```python
from build123d import *

# Parameters (mm, degrees)
BOSS_EXTRUDE1_DEPTH     = 90
BOSS_EXTRUDE2_START     = -30
SKETCH2_3_R             = 12.5
BOSS_EXTRUDE2_DEPTH     = 60
EXTRUDE_THIN1_DEPTH     = 115
SKETCH5_W               = 50
SKETCH5_H               = 20
BOSS_EXTRUDE3_DEPTH     = 230
CUT_EXTRUDE2_DEPTH      = 315.682379551
CUT_EXTRUDE2_DEPTH_BACK = 315.682379551
SKETCH5_3_R             = 5
CUT_EXTRUDE1_START      = -30
CUT_EXTRUDE1_OUTLINE_R  = 8.5
CUT_EXTRUDE1_DEPTH      = 120
RIB1_START              = -2.5
RIB1_DEPTH              = 5
FILLET1_R               = 10


# Read off the part's stored shape, not the designer's step: Cut-Extrude1, Rib1
with BuildPart() as part:
    # Sketch2 → Boss-Extrude1 (new body)
    with BuildSketch(Plane(origin=(0, 0, 0), x_dir=(1, 0, 0), z_dir=(0, 1, 0))):
        with BuildLine():
            Line((42.074338973, 6), (47.5, 6))
            Line((47.5, 6), (47.5, -6))
            Line((47.5, -6), (42.074338973, -6))
            ThreePointArc((42.074338973, -6), (-42.5, 0), (42.074338973, 6))
        make_face()
    extrude(amount=BOSS_EXTRUDE1_DEPTH)



with BuildPart() as body_2:
    # Sketch2<3> → Boss-Extrude2 (new body)
    with BuildSketch(Plane(origin=(0, 0, 0), x_dir=(1, 0, 0), z_dir=(0, 1, 0)).offset(BOSS_EXTRUDE2_START)):
        with Locations(Location((170, 0, 0), (0, 0, 270))):
            Circle(SKETCH2_3_R)
    extrude(amount=BOSS_EXTRUDE2_DEPTH)


with BuildPart() as part_1:
    add(part.part)

    add(body_2.part)  # Extrude-Thin1 merges body 2
    # Sketch3 → Extrude-Thin1 (add, symmetric)
    with BuildSketch(Plane.XY):
        Polygon((-42.5, 0), (94.247392222, 0), (130, -30), (182.5, -30), (182.5, -24), (132.183821406, -24), (96.431213628, 6), (-42.5, 6), align=None)
    extrude(amount=EXTRUDE_THIN1_DEPTH, both=True)

    # Sketch5 → Boss-Extrude3 (add)
    with BuildSketch(Plane.XY.offset(115)):
        with Locations((170, -20)):
            Rectangle(SKETCH5_W, SKETCH5_H)
    extrude(amount=-BOSS_EXTRUDE3_DEPTH)

    # Sketch5<3> → Cut-Extrude2 (cut, two sides: drawn at the far end of the back side and taken through both)
    with BuildSketch(Plane.XY.offset(115).offset(-CUT_EXTRUDE2_DEPTH_BACK)):
        with Locations((155, -20)):
            Circle(SKETCH5_3_R)
    extrude(amount=CUT_EXTRUDE2_DEPTH + CUT_EXTRUDE2_DEPTH_BACK, mode=Mode.SUBTRACT)

    # Cut-Extrude1 outline → Cut-Extrude1 (cut)
    with BuildSketch(Plane(origin=(0, 0, 0), x_dir=(1, 0, 0), z_dir=(0, 1, 0)).offset(CUT_EXTRUDE1_START)):
        with BuildLine():
            ThreePointArc((-42.5, 2.03e-07), (-27.271780209, 32.596012091), (7.5, 41.833001327))
            Line((7.5, 41.833001327), (145, 17.181411259))
            Line((145, 17.181411259), (145, 115))
            Line((145, 115), (-42.5, 115))
            Line((-42.5, 115), (-42.5, 2.03e-07))
        make_face()
        with BuildLine():
            Line((145, 115), (145, 17.181411259))
            Line((145, 17.181411259), (172.205882353, 12.30382392))
            ThreePointArc((172.205882353, 12.30382392), (179.587062361, 8.021111849), (182.5, 0))
            ThreePointArc((182.5, 0), (179.587062361, -8.021111849), (172.205882353, -12.30382392))
            Line((172.205882353, -12.30382392), (145, -17.181411259))
            Line((145, -17.181411259), (145, -115))
            Line((145, -115), (195, -115))
            Line((195, -115), (195, 115))
            Line((195, 115), (145, 115))
        make_face()
        with BuildLine():
            ThreePointArc((7.5, -41.833001327), (-27.271780365, -32.596011961), (-42.5, 2.03e-07))
            Line((-42.5, 2.03e-07), (-42.5, -115))
            Line((-42.5, -115), (145, -115))
            Line((145, -115), (145, -17.181411259))
            Line((145, -17.181411259), (7.5, -41.833001327))
        make_face()
        with BuildLine():
            Line((44.5, 3), (38.382938918, 3))
            ThreePointArc((38.382938918, 3), (-38.5, 0), (38.382938918, -3))
            Line((38.382938918, -3), (44.5, -3))
            Line((44.5, -3), (44.5, 3))
        make_face()
        with Locations((170, 0)):
            Circle(CUT_EXTRUDE1_OUTLINE_R)
    extrude(amount=CUT_EXTRUDE1_DEPTH, mode=Mode.SUBTRACT)

    # Rib1 outline → Rib1 (add)
    with BuildSketch(Plane.XY.offset(RIB1_START)):
        Polygon((151.838214056, 30), (80.3329985, 90), (47.5, 90), (47.5, 6), (96.431213628, 6), (132.183821406, -24), (145, -24), (145, -10), (159, -10), (159, 30), align=None)
    extrude(amount=RIB1_DEPTH)

    # Fillet1
    fillet1_edges = [part_1.edges().sort_by_distance(p)[0] for p in [
        (145, -10, 9.84070563),
        (132.183821406, -24, -10.989575378),
        (96.431213628, 6, -14.194515854),
        (151.838214056, 30, 0),
        (80.3329985, 90, 0),
        (145, -10, -9.84070563),
        (94.247392222, 0, 0),
        (96.431213628, 6, 14.194515854),
        (132.183821406, -24, 10.989575378),
        (130, -30, 0),
    ]]
    fillet(fillet1_edges, radius=FILLET1_R)


solid = part_1.part
```
Source: CAD feature listing. Evaluate the final solid. Frame: model axes, mm. A direction names the side the tool comes from. Give positions to 0.01 mm unless a question says otherwise; leave off trailing zeros. Order: outer loops, then holes, each group sorted by start corner. A loop starts at its lowest first (then second) coordinate and runs counter-clockwise, first axis right, second up. Notation, with made-up numbers: (68, 31.5) -> (101, 31.5) arc R14 ccw to (101, 40.5) -> close; hole circle Ø3 at (3.5, 21). An arc over 180 degrees is marked (long way). Use a Markdown table: item, result.
Q1. Section B-B (y = 26). Return the cut outline in (x, z).
A:
| item | result |
|---|---|
| outline | (42.07, -6) -> (47.5, -6) -> (47.5, -2.5) -> (157.75, -2.5) arc R12.5 ccw (long way) to (157.75, 2.5) -> (47.5, 2.5) -> (47.5, 6) -> (42.07, 6) arc R42.5 ccw (long way) to start; hole (38.38, -3) -> (44.5, -3) -> (44.5, 3) -> (38.38, 3) arc R38.5 ccw (long way) to start; hole circle Ø17 at (170, 0) |
Q2. Section A-A (z = 0). Return the cut outline in (x, y), and give its area (3 significant figures).
A:
| item | result |
|---|---|
| outline | (-42.5, 0) -> (-38.5, 0) -> (-38.5, 90) -> (-42.5, 90) -> close; (44.5, 0) -> (90.61, 0) arc R10 cw to (97.04, -2.34) -> (127.21, -27.66) arc R10 ccw to (133.64, -30) -> (161.5, -30) -> (161.5, 30) -> (155.48, 30) arc R10 cw to (149.05, 32.34) -> (83.12, 87.66) arc R10 ccw to (76.69, 90) -> (44.5, 90) -> close; (178.5, -30) -> (182.5, -30) -> (182.5, 30) -> (178.5, 30) -> close; hole circle Ø10 at (155, -20) |
| area | 9,810 mm^2 |
Q3. Access query for faces 1 (the face through (41, 44, -3)), 2 (the face through (140, -24, 11)), 3 (the face through (114.52, -9.18, -13.78)). Directions: +Z, -Z, +X, -X, +Y, -Y. A direction counts if a zero-diameter tool reaches every point of the face in a straight line with its end or side. Return the directions, or none.
A:
| item | result |
|---|---|
| face 1 | +Y, -Y |
| face 2 | +Z, +Y |
| face 3 | -Z, +Y |
Q4. Section D-D (z = -31). Return the cut outline in (x, y), and give its area (3 significant figures).
A:
| item | result |
|---|---|
| outline | (-29.07, 0) -> (-22.83, 0) -> (-22.83, 90) -> (-29.07, 90) -> close; (22.83, 0) -> (67.92, 0) -> (67.92, 6) -> (29.07, 6) -> (29.07, 90) -> (22.83, 90) -> close |
| area | 1,360 mm^2 |
Q5. Material intervals for line 1 (X direction, y = 0.5, z = 0); line 2 (Z direction, x = 170, y = 6); line 3 (X direction, y = -23, z = 2), sorted ascending. Write a range as [from, to].
A:
| item | result |
|---|---|
| line 1 | [-42.5, -38.5], [44.5, 161.5], [178.5, 182.5] |
| line 2 | [-12.5, -8.5], [8.5, 12.5] |
| line 3 | [121.66, 151], [159, 161.74], [178.26, 182.34] |
Q6. Section C-C (x = 0). Return the cut outline in (y, z), and give its area (3 significant figures).
A:
| item | result |
|---|---|
| outline | (0, -42.5) -> (90, -42.5) -> (90, -38.5) -> (0, -38.5) -> close; (0, 38.5) -> (90, 38.5) -> (90, 42.5) -> (0, 42.5) -> close |
| area | 720 mm^2 |
Q7. Pull-direction query (Z, two-part tool) for faces 4 (the face through (-38.465, 44.37, -1.651)), 5 (the face through (96.2, 5.4, 14.4)), 6 (the face through (102, 34, -2.5)); classes: +Z half, -Z half, draft (parallel to the pull), parting line (faces both ways), or undercut.
A:
| item | result |
|---|---|
| face 4 | undercut |
| face 5 | draft |
| face 6 | -Z half |
Q8. First-contact query: P1, Ø3, axis at x = 142.5, z = 9, coming from the +Y side; P2, Ø1, axis at x = 79.5, y = 25.5, coming from the -Z side; P3, Ø10.5, axis at x = 165, z = -6.5, coming from the +Y side; P4, Ø6, axis at x = 155, y = -20, coming from the -Z side. Flat tips, straight axial feed; report the tip coordinate or a pass-through.
A:
| item | result |
|---|---|
| P1 | y = -24 |
| P2 | z = -2.5 |
| P3 | y = 30 |
| P4 | through |
